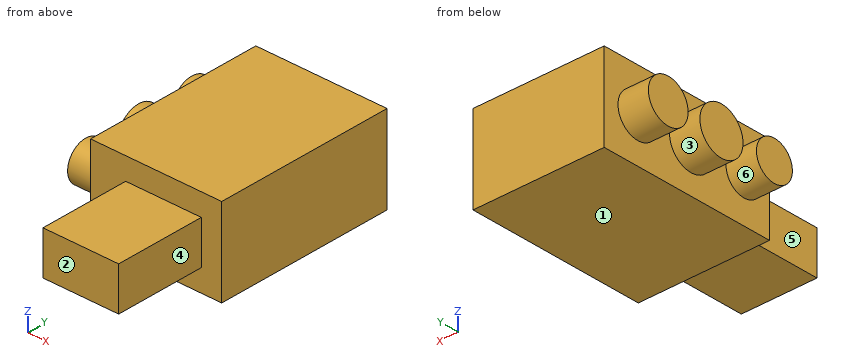
from build123d import *

# Parameters (mm, degrees)
F0_W      = 151.8585681915
F0_H      = 72.1951127052
F1_DEPTH  = 150
F2_W      = 269.2821621895
F2_H      = 145.881652832
F3_DEPTH  = 300
F4_R      = 39.1105364466
F4_R_2    = 36.046178771
F4_R_3    = 32.629936561
F6_DEPTH  = 25.4
F7_DEPTH  = 50
F8_DEPTH  = 25.4
F9_DEPTH  = 25.4
F5_W      = 269.2821621895
F5_H      = 300
F10_DEPTH = 25.4
F11_DEPTH = 25.4


with BuildPart() as f1:
    # F0 (on Front) → F1 (new body)
    with BuildSketch(Plane.XZ):
        Rectangle(F0_W, F0_H)
    extrude(amount=F1_DEPTH)

    # F2 (on face) → F3 (join)
    with BuildSketch(Plane(origin=(0, 0, 0), x_dir=(-1, 0, 0), z_dir=(0, 1, 0))):
        Rectangle(F2_W, F2_H)
    extrude(amount=F3_DEPTH)

    # F4 (on face) → F6 (join)
    with BuildSketch(Plane(origin=(-134.6410810947, 0, 0), x_dir=(0, -1, 0), z_dir=(-1, 0, 0))):
        with Locations((-142.3476338387, 0)):
            Circle(F4_R)
        with Locations((-238.8992160559, 0)):
            Circle(F4_R_2)
        with Locations((-46.2152846158, 0)):
            Circle(F4_R_3)
    extrude(amount=F6_DEPTH)

    # F7 (cut): a face of the model
    f7_faces = [f1.faces().sort_by_distance(p)[0] for p in [
        (134.6410810947, 150, 0),
    ]]
    extrude(f7_faces, amount=-F7_DEPTH, mode=Mode.SUBTRACT)

    # F8 (cut): a face of the model
    f8_faces = [f1.faces().sort_by_distance(p)[0] for p in [
        (75.9292840958, -75, 0),
    ]]
    extrude(f8_faces, amount=-F8_DEPTH, mode=Mode.SUBTRACT)

    # F9 (add): faces of the model
    f9_faces = [f1.faces().sort_by_distance(p)[0] for p in [
        (-160.0410810947, 238.8992160559, 0),
        (-160.0410810947, 142.3476338387, 0),
        (-160.0410810947, 46.2152846158, 0),
    ]]
    extrude(f9_faces, amount=F9_DEPTH)

    # F5 (on face) → F10 (cut)
    with BuildSketch(Plane.XY.offset(72.940826416)):
        with Locations((0, 150)):
            Rectangle(F5_W, F5_H)
    extrude(amount=-F10_DEPTH, mode=Mode.SUBTRACT)

    # F11 (add): a face of the model
    f11_faces = [f1.faces().sort_by_distance(p)[0] for p in [
        (-25, 150, 47.540826416),
    ]]
    extrude(f11_faces, amount=F11_DEPTH)


solid = f1.part
Can you work these out from the model? Positions are in its coordinate system, mm. Face numbers are marked on the shaded views. A direction names the side the tool comes from. Coordinates: 2 decimals unless noted, no trailing zeros. Write each loop counter-clockwise with the first axis right and the second up, starting at its lowest first coordinate (ties: lowest second). Pieces come first, ordered by that corner, then holes. Notation, with made-up numbers: (61.25, 25) - (112.25, 25) arc R25 ccw to (112.25, 40) - close; hole circle Ø7 at (28, 29). An arc over 180 degrees is marked (long way). Return JSON: item names as keys, results as strings. Group by question number.
Item 1: If we section it at C-C (x = -149): Write out the boundary of the cut face in (y, z).
Item 2: Please list where these lines run through material, in increasing order: probe 1 along Y at (x, z) = (-87, 14.5); probe 2 along Z at (x, y) = (-22.5, -84); probe 3 along X at (y, z) = (91.5, -18).
Item 3: We'd pull the mould along Y, two halves only. Please class the marked faces 1, 2 and 3: pulls with the +Y half, pulls with the -Y half, needs draft (parallel to the pull), parting line crosses it, or undercut.
Item 4: I'm going to push flat-ended pins straight in: pin 1 Ø3 at (x, y) = (-72, -43) entering from +Z; pin 2 Ø21.5 at (y, z) = (-78.5, -16.5) entering from -X. Where does each tip first touch, or does it pass through?
Item 5: If we section it at D-D (y = -106): Write out the boundary of the cut face in (x, z).
Item 6: If we section it at B-B (z = 0): Write out the boundary of the cut face in (x, y), then the cut area to 3 significant figures.
Item 7: Which directions (+Z, -Z, +X, -X, +Y, -Y) give clear straight access to the entire face, cutting with the end or side of a thin tool? Please do the marked faces 4, 5 and 6.
Item 8: If we section it at A-A (x = 34): Write out the boundary of the cut face in (y, z), then the cut area to 3 significant figures.
Return value:
{
 "1": {"outline": "circle Ø65.26 at (46.22, 0); circle Ø78.22 at (142.35, 0); circle Ø72.09 at (238.9, 0)"},
 "2": {"probe 1": "y = 0 to 300", "probe 2": "z = -36.1 to 36.1", "probe 3": "x = -134.64 to 84.64"},
 "3": {"face 1": "needs draft", "face 2": "pulls with the -Y half", "face 3": "undercut"},
 "4": {"pin 1": "stops at z = 36.1", "pin 2": "stops at x = -75.93"},
 "5": {"outline": "(-75.93, -36.1) - (50.53, -36.1) - (50.53, 36.1) - (-75.93, 36.1) - close"},
 "6": {"outline": "(-185.44, 13.59) - (-134.64, 13.59) - (-134.64, 0) - (-75.93, 0) - (-75.93, -150) - (50.53, -150) - (50.53, 0) - (84.64, 0) - (84.64, 300) - (-134.64, 300) - (-134.64, 274.95) - (-185.44, 274.95) - (-185.44, 202.85) - (-134.64, 202.85) - (-134.64, 181.46) - (-185.44, 181.46) - (-185.44, 103.24) - (-134.64, 103.24) - (-134.64, 78.85) - (-185.44, 78.85) - close", "area": "95,700 mm^2"},
 "7": {"face 4": "+Z, -Z, +X, -Y", "face 5": "+Z, -Z, -X, -Y", "face 6": "-X"},
 "8": {"outline": "(-150, -36.1) - (0, -36.1) - (0, -72.94) - (300, -72.94) - (300, 72.94) - (0, 72.94) - (0, 36.1) - (-150, 36.1) - close", "area": "54,600 mm^2"}
}
